Answer from the drawing. Dimensions are ordinates in mm from the lowest x, y and z of the part. A direction names the side the tool comes from. Coordinates: 2 decimals unless noted, no trailing zeros. Loops run counter-clockwise (first coordinate to the right, second up) from the corner with the lowest first, then second, coordinate; pieces in that order, holes last. Notation, with made-up numbers: (-28.5, 40) - (11.5, 40) arc R12 cw to (11.5, 55) - close; hole circle Ø8 at (58, -19). An arc over 180 degrees is marked (long way). Use one line per item in the form item = value. Start each with the question number.
1) A cutting plane is placed at A-A (x = 16.75). State how many separate pieces and enclosed holes the cut face has, and give its area (3 significant figures).
2) Each of these flat-tipped pins is pushed along its axis until it touches: P1, Ø4, axis at x = 6, z = 8, coming from the -Y side; P2, Ø3, axis at x = 7, y = 4.5, coming from the -Z side; P3, Ø5, axis at y = 5.5, z = 6, coming from the +X side; P4, Ø3, axis at x = 28, y = 7, coming from the -Z side. Where does it stop, or does it pass through?
3) Consider line 1 (Z direction, x = 17, y = 2.5); line 2 (X direction, y = 3, z = 16.75); line 3 (Z direction, x = 15.5, y = 0.5). Determine where each line is inside the solid, lowest interval first.
4) The mould has two halves that part along Z. Classify the marked faces 3, 4 and 5: released by +Z, released by -Z, zero draft, split by the parting line, or undercut.
5) Which of the six approach directions +Z, -Z, +X, -X, +Y, -Y give full straight-line access (tool end or side, diameter ignored) to the marked faces 1 and 2?
6) A cutting plane is placed at B-B (y = 5). Give the vertices of the cut face in (x, z), and give its area (3 significant figures).
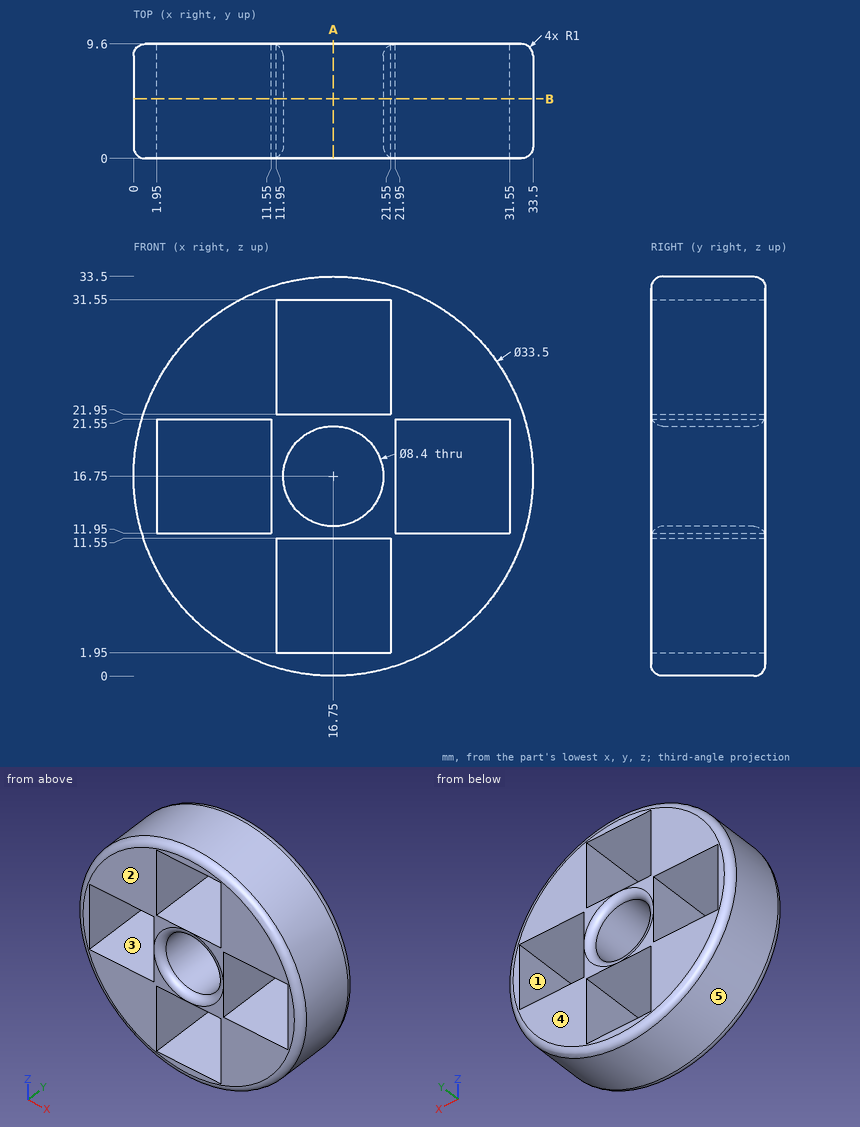
Found:
q1.separate_pieces = 4
q1.enclosed_holes = 0
q1.area = 54.9 mm^2
q2.P1 = 0
q2.P2 = 2.17
q2.P3 = 31.33
q2.P4 = 3.13
q3.line_1 = 0 to 1.95, 11.55 to 12.56, 20.94 to 21.95, 31.55 to 33.5
q3.line_2 = 0 to 1.95, 11.55 to 12.55, 20.95 to 21.95, 31.55 to 33.5
q3.line_3 = 0.18 to 1.95, 11.55 to 12.6, 20.9 to 21.95, 31.55 to 33.32
q4.face_3 = undercut
q4.face_4 = zero draft
q4.face_5 = split by the parting line
q5.face_1 = +Y, -Y
q5.face_2 = +Z, -Z, +X, -X, -Y
q6.outline = circle Ø33.5 at (16.75, 16.75); hole (1.95, 11.95) - (11.55, 11.95) - (11.55, 21.55) - (1.95, 21.55) - close; hole (11.95, 1.95) - (21.55, 1.95) - (21.55, 11.55) - (11.95, 11.55) - close; hole (11.95, 21.95) - (21.55, 21.95) - (21.55, 31.55) - (11.95, 31.55) - close; hole circle Ø8.4 at (16.75, 16.75); hole (21.95, 11.95) - (31.55, 11.95) - (31.55, 21.55) - (21.95, 21.55) - close
q6.area = 457 mm^2
